Autodesk Inventor part; units mm, degrees
ref_plane "YZ Plane" through (0, 0, 0) normal (1, 0, 0) x (0, 1, 0)
ref_plane "XZ Plane" through (0, 0, 0) normal (0, 1, 0) x (-1, 0, 0)
ref_plane "XY Plane" through (0, 0, 0) normal (0, 0, 1) x (1, 0, 0)
sketch "Sketch1" plane through (0, 0, 0) normal (0, 1, 0) x (-1, 0, 0)
  line L0 (-5.4846, 0) -> (-2.7423, 4.7498)
  line L1 (-2.7423, 4.7498) -> (2.7423, 4.7498)
  line L2 (2.7423, 4.7498) -> (5.4846, 0)
  line L3 (5.4846, 0) -> (2.7423, -4.7498)
  line L4 (2.7423, -4.7498) -> (-2.7423, -4.7498)
  line L5 (-2.7423, -4.7498) -> (-5.4846, 0)
  line L6 (-2.5957, -4.4958) -> (2.5957, -4.4958)
  line L7 (2.5957, -4.4958) -> (5.1913, 0)
  line L8 (5.1913, 0) -> (2.5957, 4.4958)
  line L9 (2.5957, 4.4958) -> (-2.5957, 4.4958)
  line L10 (-2.5957, 4.4958) -> (-5.1913, 0)
  line L11 (-5.1913, 0) -> (-2.5957, -4.4958)
  point P0 (0, 0)
  point P1 (0, 0)
  dimension "d0" = 9.4996
  dimension "d1" = 0.254
extrude "Extrusion1" add sketch "Sketch1" along normal blind 6.35 contours L11 L10 L9 L8 L7 L6
sketch "Sketch2" plane through (0, 6.35, 0) normal (0, 1, 0) x (1, 0, 0)
  circle A0 centre (0, 0) radius 6.35
  line L0 (1.6002, -1.6002) -> (-1.6002, -1.6002)
  line L1 (-1.6002, -1.6002) -> (-1.6002, 1.6002)
  line L2 (-1.6002, 1.6002) -> (1.6002, 1.6002)
  line L3 (1.6002, 1.6002) -> (1.6002, -1.6002)
  line L4 (1.6002, -1.6002) -> (-1.6002, 1.6002) construction
  line L5 (-1.6002, -1.6002) -> (1.6002, 1.6002) construction
  dimension "d4" = 12.7
  dimension "d5" = 3.2004
  dimension "d6" = 3.2004
extrude "Extrusion2" add sketch "Sketch2" along normal blind 3.175
sketch "Sketch3" plane through (0, 9.525, 0) normal (0, 1, 0) x (1, 0, 0)
  line L0 (-1.6002, -1.6002) -> (-1.6002, 1.6002)
  line L1 (-1.6002, 1.6002) -> (-1.6002, -1.6002)
  line L2 (-1.6002, -1.6002) -> (1.6002, -1.6002)
  line L3 (1.6002, -1.6002) -> (1.6002, 1.6002)
  line L4 (1.6002, 1.6002) -> (-1.6002, 1.6002)
  point P0 (0, 0)
extrude "Extrusion3" cut sketch "Sketch3" against normal through all
fillet "Fillet1" radius 0.5292 4 edges at (0, 9.525, -1.6002) (1.6002, 9.525, 0) (-1.6002, 9.525, 0) (0, 9.525, 1.6002)
properties part number "Flex Wheel Connector"
Input: part model. Units: mm. Frame: model coordinates. A direction names the side the tool comes from. Give positions to 0.01 mm unless a question says otherwise; leave off trailing zeros. Write each loop counter-clockwise with the first axis right and the second up, starting at its lowest first coordinate (ties: lowest second). Pieces come first, ordered by that corner, then holes. Notation, with made-up numbers: (45.5, -29.5) - (51.5, -29.5) arc R12 cw to (51.5, -9.5) - close; hole circle Ø4 at (29, 73.25). An arc over 180 degrees is marked (long way). Write item = value, one per line. Start each with the question number.
1. Section query A-A, the plane y = 1. Output: boundary loops of the cut face in (x, z).
2. Mould query, pull axis Z, two halves, no side actions, for faces 4 (the flat face through (0, 5, -1.6)), 5 (the flat face through (0, 3, -4.496)), 6 (the flat face through (0, 3, 4.496)). Classes: released by +Z, released by -Z, zero draft, split by the parting line, or undercut.
3. Ray query, L1, parallel to X at y = 8.75, z = 0; L2, parallel to Z at x = 0.25, y = 4.5; L3, parallel to X at y = 3.75, z = -0.75. Return the intervals inside material, ascending.
4. Section query B-B, the plane x = 0. Output: boundary loops of the cut face in (y, z) (3 decimals), then the cut area to 3 significant figures.
5. First-contact query: pin 1 Ø2.5 at (x, y) = (1, 2.5) entering from +Z; pin 2 Ø3 at (y, z) = (3.5, -2.5) entering from +X; pin 3 Ø4 at (x, y) = (1, 2.5) entering from -Z; pin 4 Ø4 at (x, z) = (0.5, 2) entering from -Y. Flat tips, straight axial feed; report the tip coordinate or a pass-through.
6. Access query for faces 1 (the flat face through (1.6, 5, 0)), 2 (the flat face through (3.875, 3.131, 2.279)), 3 (the flat face through (-4.3, 6.35, 1.9)). Directions: +Z, -Z, +X, -X, +Y, -Y. A direction counts if a zero-diameter tool reaches every point of the face in a straight line with its end or side. Return the directions, or none.
7. Section query D-D, the plane x = 5. Output: boundary loops of the cut face in (y, z) (3 decimals).
8. Section query C-C, the plane z = 0.5. Output: boundary loops of the cut face in (x, y) (3 decimals).
Check sheet entries:
q1.outline = (-5.19, 0) - (-2.6, -4.5) - (2.6, -4.5) - (5.19, 0) - (2.6, 4.5) - (-2.6, 4.5) - close; hole (-1.6, -1.6) - (1.6, -1.6) - (1.6, 1.6) - (-1.6, 1.6) - close
q2.face_4 = undercut
q2.face_5 = released by -Z
q2.face_6 = released by +Z
q3.L1 = -6.35 to -1.6, 1.6 to 6.35
q3.L2 = -4.5 to -1.6, 1.6 to 4.5
q3.L3 = -4.76 to -1.6, 1.6 to 4.76
q4.outline = (0, -4.496) - (6.35, -4.496) - (6.35, -6.35) - (9.525, -6.35) - (9.525, -2.129) arc R0.529 ccw to (8.996, -1.6) - (0, -1.6) - close; (0, 1.6) - (8.996, 1.6) arc R0.529 ccw to (9.525, 2.129) - (9.525, 6.35) - (6.35, 6.35) - (6.35, 4.496) - (0, 4.496) - close
q4.area = 66.8 mm2
q5.pin_1 = 4.5
q5.pin_2 = 4.61
q5.pin_3 = -4.5
q5.pin_4 = 0
q6.face_1 = +Y, -Y
q6.face_2 = +Z, +X, -Y
q6.face_3 = -Y
q7.outline = (0, -0.331) - (6.35, -0.331) - (6.35, -3.914) - (9.525, -3.914) - (9.525, 3.914) - (6.35, 3.914) - (6.35, 0.331) - (0, 0.331) - close
q8.outline = (-6.33, 6.35) - (-4.903, 6.35) - (-4.903, 0) - (-1.6, 0) - (-1.6, 8.996) arc R0.529 ccw to (-2.129, 9.525) - (-6.33, 9.525) - close; (1.6, 0) - (4.903, 0) - (4.903, 6.35) - (6.33, 6.35) - (6.33, 9.525) - (2.129, 9.525) arc R0.529 ccw to (1.6, 8.996) - close
